The listing builds one solid part. Answer for the finished solid, in the listing's coordinates (mm). Round coordinates to 2 decimals unless told otherwise and drop trailing zeros. Loops run counter-clockwise (first coordinate to the right, second up) from the corner with the lowest first, then second, coordinate; pieces in that order, holes last. Notation, with made-up numbers: M -11,56.5 L -5,56.5 A14 cw -5,70.5 Z; hole C 51,74 d2. An arc over 180 degrees is marked long. Answer as a JSON object with one key per item and string values.
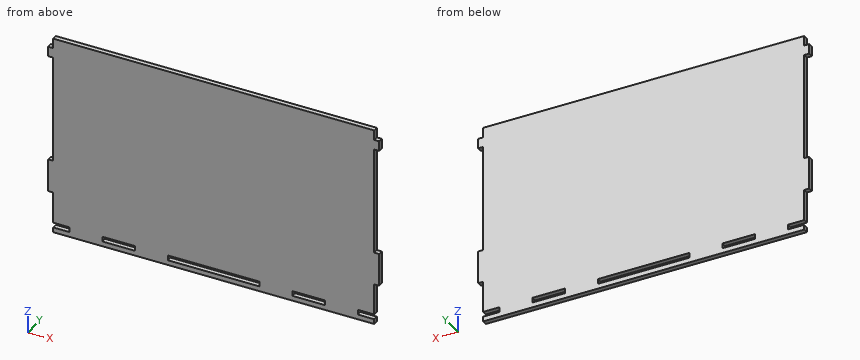
```python
from build123d import *

# Parameters (mm, degrees)
F0_W     = 20
F0_H     = 3
F0_W_2   = 56
F1_DEPTH = 1.5


with BuildPart() as f1:
    # F0 (on Front) → F1 (new body, symmetric)
    with BuildSketch(Plane.XZ):
        Polygon((-98, -56.5), (-88, -56.5), (-88, -59.5), (-98, -59.5), (-98, -62.5), (0, -62.5), (98, -62.5), (98, -59.5), (88, -59.5), (88, -56.5), (98, -56.5), (98, -37.5), (101, -37.5), (101, -17.5), (98, -17.5), (98, 47.5), (101, 47.5), (101, 53.5), (98, 53.5), (98, 59.5), (0, 59.5), (-98, 59.5), (-98, 53.5), (-101, 53.5), (-101, 47.5), (-98, 47.5), (-98, -17.5), (-101, -17.5), (-101, -37.5), (-98, -37.5), align=None)
        with Locations((-58, -58)):
            Rectangle(F0_W, F0_H, mode=Mode.SUBTRACT)
        with Locations((0, -58)):
            Rectangle(F0_W_2, F0_H, mode=Mode.SUBTRACT)
        with Locations((58, -58)):
            Rectangle(F0_W, F0_H, mode=Mode.SUBTRACT)
    extrude(amount=F1_DEPTH, both=True)


solid = f1.part
```
Item 1: Straight lines are drawn through the part: line 1 (Z direction, x = -89.5, y = -0.6); line 2 (X direction, y = 0.15, z = 44.5). For each, find the intervals that lie inside material, in ascending order.
Values follow:
{"line 1": "-62.5 to -59.5, -56.5 to 59.5", "line 2": "-98 to 98"}
Item 2: The part is cut by section A-A (x = 9). Give the vertices of the cut face in (y, z).
Values follow:
{"outline": "M -1.5,-62.5 L 1.5,-62.5 L 1.5,-59.5 L -1.5,-59.5 Z; M -1.5,-56.5 L 1.5,-56.5 L 1.5,59.5 L -1.5,59.5 Z"}
Item 3: The part is cut by section C-C (y = -0.65). Give the number of separate pieces and of enclosed holes in the cut face, then the cut area to 3 significant figures.
Values follow:
{"separate pieces": "1", "enclosed holes": "3", "area": "23,700 mm^2"}
Item 4: The part is cut by section B-B (z = 38). Give the vertices of the cut face in (x, y), then the cut area to 3 significant figures.
Values follow:
{"outline": "M -98,-1.5 L 98,-1.5 L 98,1.5 L -98,1.5 Z", "area": "588 mm^2"}
Item 5: Flat-ended cylindrical pins translate along their axes: P1, Ø1.5, axis at y = -0.5, z = -60.5, coming from the +X side; P2, Ø1.5, axis at y = 0.5, z = -58, coming from the +X side; P3, Ø0.9, axis at y = 0.5, z = -58.5, coming from the -X side. Find the tip coordinate at first contact, or state that the pin passes through.
Values follow:
{"P1": "x = 98", "P2": "x = 88", "P3": "x = -88"}
